Build history of the part. All positions in model axes, mm. Face numbers are marked on the shaded views. A direction names the side the tool comes from. Round coordinates to 2 decimals unless told otherwise and drop trailing zeros. Order: outer loops, then holes, each group sorted by start corner. A loop starts at its lowest first (then second) coordinate and runs counter-clockwise, first axis right, second up. Notation, with made-up numbers: (32, 85.5) -> (67, 85.5) arc R20 ccw to (67, 95.5) -> close; hole circle Ø5 at (-10, -34.5). An arc over 180 degrees is marked (long way). Answer as CSV lines item,"result". Start each with the question number.
```python
from build123d import *

# Parameters (mm, degrees)
F1_DEPTH = 63.5
F0_W     = 16.068018
F0_H     = 19.05
F2_DEPTH = 25.4
F3_DEPTH = 7.9375
F5_R     = 12.7


with BuildPart() as f1:
    # F0 (on Front) → F1 (new body, symmetric)
    with BuildSketch(Plane.XZ):
        Polygon((22.225, 9.525), (-41.275, 9.525), (-41.275, -9.525), (41.275, -9.525), (41.275, 9.525), align=None)
    extrude(amount=F1_DEPTH, both=True)

    # F0 (on Front) → F2 (join, symmetric)
    with BuildSketch(Plane.XZ):
        with BuildLine():
            Line((22.225, 35.372035), (22.225, 9.525))
            Line((22.225, 9.525), (41.275, 9.525))
            Line((41.275, 9.525), (41.275, 35.372035))
            ThreePointArc((41.275, 35.372035), (48.714488, 53.332548), (66.675, 60.772035))
            Line((66.675, 60.772035), (70.067601, 60.772035))
            Line((70.067601, 60.772035), (70.067601, 79.822035))
            Line((70.067601, 79.822035), (66.675, 79.822035))
            add(Edge.make_bspline(
                [(66.274157, 79.820228), (66.407695, 79.820948), (66.541309, 79.82155), (66.675, 79.822035)],
                knots=[128.53936, 128.53936, 128.53936, 128.53936, 128.8211, 128.8211, 128.8211, 128.8211], degree=3))
            ThreePointArc((66.274157, 79.820228), (35.102702, 66.660891), (22.225, 35.372035))
        make_face()
        with Locations((78.10161, 70.297035)):
            Rectangle(F0_W, F0_H)
    extrude(amount=F2_DEPTH, both=True)

    # F0 (on Front) → F3 (join, symmetric)
    with BuildSketch(Plane.XZ):
        with BuildLine():
            add(Edge.make_bspline(
                [(-41.275, 9.525), (-39.656203, 54.754084), (5.349448, 79.491852), (66.274157, 79.820228)],
                knots=[0, 0, 0, 0, 128.53936, 128.53936, 128.53936, 128.53936], degree=3))
            Line((-41.275, 9.525), (22.225, 9.525))
            Line((22.225, 9.525), (22.225, 35.372035))
            ThreePointArc((22.225, 35.372035), (35.102702, 66.660891), (66.274157, 79.820228))
        make_face()
    extrude(amount=F3_DEPTH, both=True)

    # F0 (on Front) → F4 (revolve)
    with BuildSketch(Plane.XZ):
        with BuildLine():
            Line((120.867601, 85.725), (95.467601, 85.725))
            Line((95.467601, 85.725), (95.467601, 71.4375))
            Line((95.467601, 71.4375), (95.467601, 71.145688))
            ThreePointArc((95.467601, 71.145688), (105.364047, 67.046446), (109.463289, 57.15))
            Line((109.463289, 57.15), (120.867601, 57.15))
            Line((120.867601, 57.15), (120.867601, 85.725))
        make_face()
    revolve(axis=Axis((95.467601, 0, 71.4375), (0, 0, -1)))

    # F5
    f5_edges = [f1.edges().sort_by_distance(p)[0] for p in [
        (-41.275, -63.5, 0),
        (41.275, -63.5, 0),
        (41.275, 63.5, 0),
        (-41.275, 63.5, 0),
    ]]
    fillet(f5_edges, radius=F5_R)


solid = f1.part
```
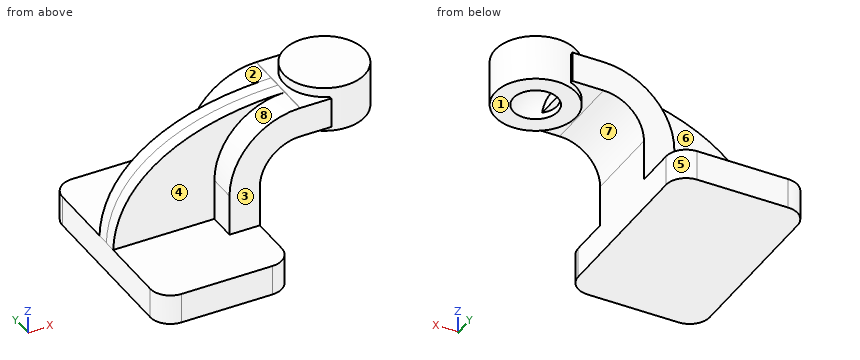
Q1. Two-plate mould, pull along X, no slides. Class the marked faces 5, 6, 7 and 8: +X half, -X half, draft (parallel to the pull), parting line (faces both ways), or undercut.
Q2. Flat gauge pins, fed straight in: pin 1 Ø1.3 at (x, y) = (84, -1.5) entering from -Z; pin 2 Ø15 at (x, y) = (85.5, -8) entering from -Z; pin 3 Ø21 at (x, z) = (24, 39.5) entering from -Y. Where does each tip first touch, or does it go through?
Q3. Slice it at A-A, the plane z = 5. Write the cut outline in (x, y) (3 decimals), plus the area to 3 significant figures.
Q4. Probe L1, parallel to Y at x = 59, z = 77; L2, parallel to Y at x = 36.5, z = 75.5; L3, parallel to Z at x = -13, y = -21.5 (3 decimals). List the from-to ranges inside material, lowest first.
Q5. Which spindle directions (+Z, -Z, +X, -X, +Y, -Y) get a long thin tool onto all of the face, cutting with end or side? Do the marked faces 1, 2, 3 and 4. Say none if no direction does.
Solutions:
1,face 5,"+X half"
1,face 6,"draft"
1,face 7,"undercut"
1,face 8,"-X half"
2,pin 1,"stops at z = 60.77"
2,pin 2,"stops at z = 57.15"
2,pin 3,"stops at y = -25.4"
3,outline,"(-41.275, -50.8) arc R12.7 ccw to (-28.575, -63.5) -> (28.575, -63.5) arc R12.7 ccw to (41.275, -50.8) -> (41.275, 50.8) arc R12.7 ccw to (28.575, 63.5) -> (-28.575, 63.5) arc R12.7 ccw to (-41.275, 50.8) -> close"
3,area,"10,300 mm2"
4,L1,"y = -25.4 to 25.4"
4,L2,"y = -7.94 to 7.94"
4,L3,"z = -9.525 to 9.525"
5,face 1,"-Z, +X, +Y, -Y"
5,face 2,"+Z, -X, +Y"
5,face 3,"+Z, +X, -X, -Y"
5,face 4,"+Z, -X, -Y"
